Could you check a few things on this model? Use its own coordinates, in mm. Round coordinates to 2 decimals unless told otherwise and drop trailing zeros. Order: outer loops, then holes, each group sorted by start corner. A loop starts at its lowest first (then second) coordinate and runs counter-clockwise, first axis right, second up.
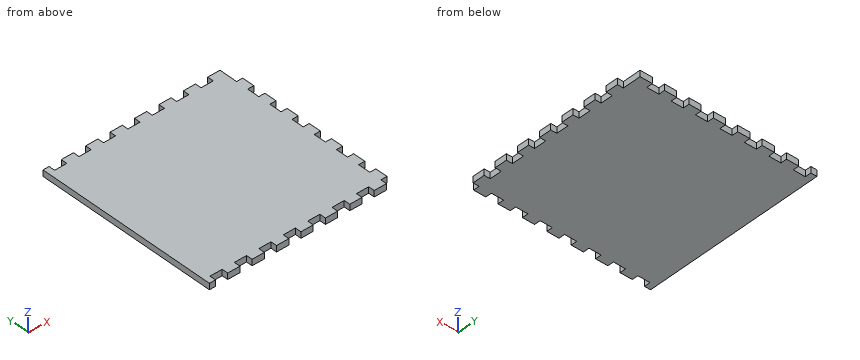
```python
from build123d import *

# Parameters (mm, degrees)
F0_W     = 300
F0_H     = 300
F1_DEPTH = 10
F2_W     = 19.925
F2_H     = 10
F2_W_2   = 10
F2_H_2   = 19.925
F3_DEPTH = 10.001


with BuildPart() as f1:
    # F0 (on Top) → F1 (new body)
    with BuildSketch(Plane.XY):
        with Locations((150, 150)):
            Rectangle(F0_W, F0_H)
    extrude(amount=F1_DEPTH)

    # F2 (on face) → F3 (cut, through all)
    with BuildSketch(Plane.XY):
        with Locations((19.9625, 5)):
            Rectangle(F2_W, F2_H)
        with Locations((59.9625, 5)):
            Rectangle(F2_W, F2_H)
        with Locations((99.9625, 5)):
            Rectangle(F2_W, F2_H)
        with Locations((139.9625, 5)):
            Rectangle(F2_W, F2_H)
        with Locations((179.9625, 5)):
            Rectangle(F2_W, F2_H)
        with Locations((219.9625, 5)):
            Rectangle(F2_W, F2_H)
        with Locations((259.9625, 5)):
            Rectangle(F2_W, F2_H)
        with Locations((299.9625, 5)):
            Rectangle(F2_W, F2_H)
        with Locations((295, 40.0375)):
            Rectangle(F2_W_2, F2_H_2)
        with Locations((295, 80.0375)):
            Rectangle(F2_W_2, F2_H_2)
        with Locations((295, 120.0375)):
            Rectangle(F2_W_2, F2_H_2)
        with Locations((295, 160.0375)):
            Rectangle(F2_W_2, F2_H_2)
        with Locations((295, 200.0375)):
            Rectangle(F2_W_2, F2_H_2)
        with Locations((295, 240.0375)):
            Rectangle(F2_W_2, F2_H_2)
        with Locations((295, 280.0375)):
            Rectangle(F2_W_2, F2_H_2)
        with Locations((295, 295)):
            Rectangle(F2_W_2, F2_H)
        with Locations((259.9625, 295)):
            Rectangle(F2_W, F2_H)
        with Locations((219.9625, 295)):
            Rectangle(F2_W, F2_H)
        with Locations((179.9625, 295)):
            Rectangle(F2_W, F2_H)
        with Locations((139.9625, 295)):
            Rectangle(F2_W, F2_H)
        with Locations((99.9625, 295)):
            Rectangle(F2_W, F2_H)
        with Locations((59.9625, 295)):
            Rectangle(F2_W, F2_H)
        with Locations((19.9625, 295)):
            Rectangle(F2_W, F2_H)
    extrude(amount=F3_DEPTH, mode=Mode.SUBTRACT)


solid = f1.part
```
Q1. Imagine slicing it at B-B, the plane x = 183. Please give me the cut outline in (y, z).
Q2. Imagine slicing it at A-A, the plane y = 73.5. Please give me the cut outline in (x, z), then the cut area to 3 significant figures.
Q3. I need wall thicknesses on L1, parallel to X at y = 239.5, z = 9.75; L2, parallel to Y at x = 188.5, z = 3.25. Which ranges of each line are inside material? Lowest first, please.
Q4. For P1, Ø3, axis at y = 293.5, z = 5, coming from the +X side; P2, Ø5, axis at x = 295.5, z = 5.5, coming from the +Y side (3 decimals); P3, Ø6, axis at x = 99.5, z = 6.5, coming from the -Y side, each with a flat end and sliding along its axis, tell me the tip position at first contact or that it passes through.
Filled in:
1. outline: (10, 0) - (290, 0) - (290, 10) - (10, 10) - close
2. outline: (0, 0) - (290, 0) - (290, 10) - (0, 10) - close
2. area: 2,900 mm2
3. L1: x = 0 to 290
3. L2: y = 10 to 290
4. P1: stops at x = 290
4. P2: stops at y = 270.075
4. P3: stops at y = 10
